Part model, mm, in its own coordinate system. Face numbers are marked on the shaded views. A direction names the side the tool comes from. Give positions to 0.01 mm unless a question says otherwise; leave off trailing zeros. Order: outer loops, then holes, each group sorted by start corner. A loop starts at its lowest first (then second) coordinate and runs counter-clockwise, first axis right, second up. Notation, with made-up numbers: M -3,30 L 27,30 A17 ccw 27,51 Z; hole C 51.25,-37 d2. An arc over 180 degrees is marked long. Write each question's results on one line, items separated by ' | '. Start each with the question number.
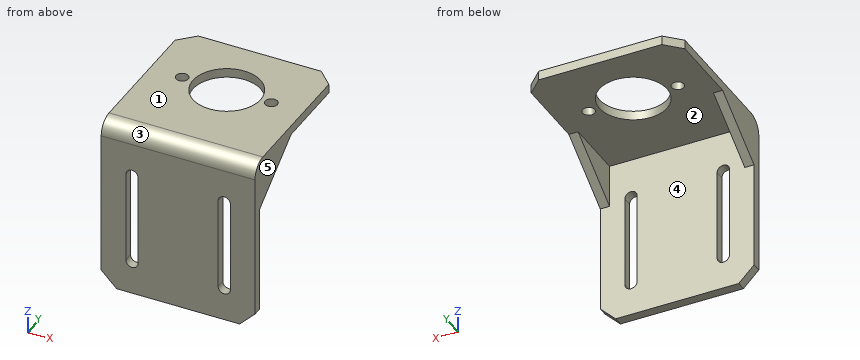
from build123d import *

# Parameters (mm, degrees)
SKETCH_1_W          = 50
SKETCH_1_H          = 52
EXTRUDE_1_DEPTH     = 3
SKETCH_2_W          = 50
SKETCH_2_H          = 3
EXTRUDE_2_DEPTH     = 54
SKETCH_3_R          = 11
SKETCH_3_R_2        = 2
CUT_EXTRUDE_1_DEPTH = 68.453687816
CHAMFER_1_SIZE      = 5
CHAMFER_2_SIZE      = 5
CUT_EXTRUDE_2_DEPTH = 80.025312401
EXTRUDE_START       = -50
EXTRUDE_3_DEPTH     = 50
CUT_EXTRUDE_START   = -3
CUT_EXTRUDE_3_DEPTH = 44
FILLET_1_R          = 5


with BuildPart() as part:
    # 草圖1 → 填料-伸長1 (new body)
    with BuildSketch(Plane.XY):
        Rectangle(SKETCH_1_W, SKETCH_1_H)
    extrude(amount=EXTRUDE_1_DEPTH)

    # 草圖2 → 填料-伸長2 (add)
    with BuildSketch(Plane(origin=(0, 0, 0), x_dir=(-1, 0, 0), z_dir=(0, 0, -1))):
        with Locations((0, -24.5)):
            Rectangle(SKETCH_2_W, SKETCH_2_H)
    extrude(amount=EXTRUDE_2_DEPTH)

    # 草圖3 → 除料-伸長1 (cut, through all)
    with BuildSketch(Plane.XY.offset(3)):
        with Locations((0, 5)):
            Circle(SKETCH_3_R)
        with Locations((14.5, 5)):
            Circle(SKETCH_3_R_2)
        with Locations((-14.5, 5)):
            Circle(SKETCH_3_R_2)
    extrude(amount=-CUT_EXTRUDE_1_DEPTH, mode=Mode.SUBTRACT)

    # 導角1
    chamfer_1_edges = [part.edges().sort_by_distance(p)[0] for p in [
        (-25, 26, 1.5),
        (25, 26, 1.5),
    ]]
    chamfer(chamfer_1_edges, length=CHAMFER_1_SIZE)

    # 導角2
    chamfer_2_edges = [part.edges().sort_by_distance(p)[0] for p in [
        (25, -24.5, -54),
        (-25, -24.5, -54),
    ]]
    chamfer(chamfer_2_edges, length=CHAMFER_2_SIZE)

    # 草圖4 → 除料-伸長2 (cut, through all)
    with BuildSketch(Plane.XZ.offset(26)):
        with BuildLine():
            Line((13, -43), (13, -13))
            ThreePointArc((13, -13), (15, -11), (17, -13))
            Line((17, -13), (17, -43))
            ThreePointArc((17, -43), (15, -45), (13, -43))
        make_face()
        with BuildLine():
            Line((-13, -43), (-13, -13))
            ThreePointArc((-13, -13), (-15, -11), (-17, -13))
            Line((-17, -13), (-17, -43))
            ThreePointArc((-17, -43), (-15, -45), (-13, -43))
        make_face()
    extrude(amount=-CUT_EXTRUDE_2_DEPTH, mode=Mode.SUBTRACT)

    # 草圖5 → 填料-伸長3 (add)
    with BuildSketch(Plane(origin=(25, 0, 0), x_dir=(0, 0, -1), z_dir=(1, 0, 0)).offset(EXTRUDE_START)):
        Polygon((0, -23), (0, -3), (14, -23), align=None)
    extrude(amount=EXTRUDE_3_DEPTH)

    # 草圖6 → 除料-伸長3 (cut)
    with BuildSketch(Plane(origin=(25, 0, 0), x_dir=(0, 0, -1), z_dir=(1, 0, 0)).offset(CUT_EXTRUDE_START)):
        Polygon((0, -3), (14, -23), (0, -23), align=None)
    extrude(amount=-CUT_EXTRUDE_3_DEPTH, mode=Mode.SUBTRACT)

    # 圓角1
    fillet_1_edges = [part.edges().sort_by_distance(p)[0] for p in [
        (0, -26, 3),
    ]]
    fillet(fillet_1_edges, radius=FILLET_1_R)


solid = part.part
(1) Saw through at D-D on x = -15. Give the cut face in (y, z).
(2) Probe L1, parallel to Z at x = 22, y = 16; L2, parallel to Y at x = -14.5, z = 1.8; L3, parallel to Y at x = -14.5, z = 0.65. List the from-to ranges inside material, lowest first.
(3) Saw through at C-C on y = -14. Give the cut face in (x, z).
(4) Saw through at A-A on z = -15. Give the cut face in (x, y), plus the area to 3 significant figures.
(5) Saw through at B-B on x = -7.5. Give the cut face in (y, z).
(6) Drop flat-ended pins along their axis: P1, Ø15, axis at x = 1.5, z = -30, coming from the +Y side; P2, Ø1.5, axis at x = -12.5, y = 14.5, coming from the -Z side. Give the stop position or say it passes through.
(7) Pull direction X, two halves, no side cores. Call the marked faces 3, 4 and 5: +X half, -X half, draft (parallel to the pull), parting line (faces both ways), or undercut.
(8) Tool access for the marked faces 1 and 2: list every direction of +Z, -Z, +X, -X, +Y, -Y with a clear straight run to the whole face (end or side of a thin tool).
Taken from the geometry:
1) outline: M -26,-54 L -23,-54 L -23,-45 L -26,-45 Z; M -26,-11 L -23,-11 L -23,0 L 3.06,0 L 3.06,3 L -21,3 A5 ccw -26,-2 Z; M 6.94,0 L 26,0 L 26,3 L 6.94,3 Z
2) L1: z = 0 to 3 | L2: y = -24.25 to 3, 7 to 26 | L3: y = -25.24 to 3, 7 to 26
3) outline: M -25,-7.7 L -22,-7.7 L -22,0 L 22,0 L 22,-7.7 L 25,-7.7 L 25,3 L -25,3 Z
4) outline: M -25,-26 L -17,-26 L -17,-23 L -25,-23 Z; M -13,-26 L 13,-26 L 13,-23 L -13,-23 Z; M 17,-26 L 25,-26 L 25,-23 L 17,-23 Z | area: 126 mm²
5) outline: M -26,-54 L -23,-54 L -23,0 L -3.05,0 L -3.05,3 L -21,3 A5 ccw -26,-2 Z; M 13.05,0 L 26,0 L 26,3 L 13.05,3 Z
6) P1: stops at y = -23 | P2: stops at z = 0
7) face 3: draft | face 4: undercut | face 5: +X half
8) face 1: +Z, +X, -X, +Y, -Y | face 2: -Z, +Y
